from build123d import *

# Parameters (mm, degrees)
MATRIZC1_COUNT = 3


with BuildPart() as part:
    # Croquis8 → Revolución4 (revolve)
    with BuildSketch(Plane.XY):
        with BuildLine():
            Line((-10, 22.912878475), (-10, 17.320508076))
            ThreePointArc((-10, 17.320508076), (-2.679491924, 10), (0, 0))
            Line((0, 0), (10, 0))
            Line((10, 0), (10, 22.912878475))
            ThreePointArc((10, 22.912878475), (0, 25), (-10, 22.912878475))
        make_face()
    revolve(axis=Axis((0, 0, 0), (1, 0, 0)))

    # Croquis3 → Revolución5 (revolve)
    with BuildSketch(Plane(origin=(0, 0, 0), x_dir=(0, 0, -1), z_dir=(1, 0, 0))):
        with BuildLine():
            Line((0, 25), (0, 34))
            ThreePointArc((0, 34), (3.968118785, 30.50401717), (1, 26.127016654))
            Line((1, 26.127016654), (1, 24.979991994))
            ThreePointArc((1, 24.979991994), (0.50010007, 24.994997498), (0, 25))
        make_face()
    revoluci_n5 = revolve(axis=Axis((0, 25, 0), (0, 1, 0)))

    # MatrizC1: Revolución5 ×3 about axis
    matrizc1_axis = Axis((0, 0, 0), (1, 0, 0))
    for i in range(1, MATRIZC1_COUNT):
        add(revoluci_n5.rotate(matrizc1_axis, i * 360 / MATRIZC1_COUNT))


solid = part.part
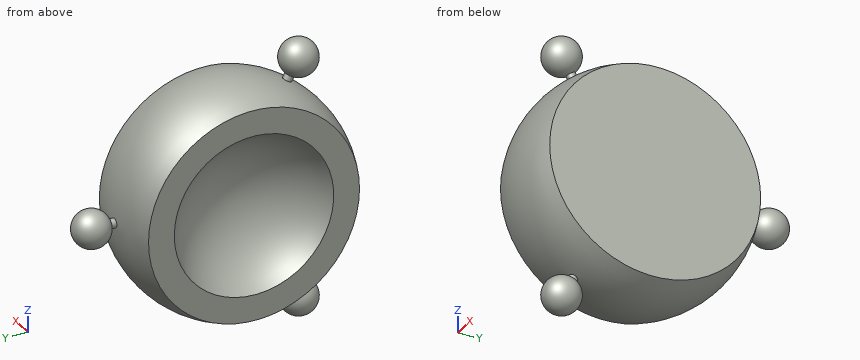
The listing builds one solid part. Answer for the finished solid, in the listing's coordinates (mm). Give positions to 0.01 mm unless a question says otherwise; leave off trailing zeros. Write each loop counter-clockwise with the first axis right and the second up, starting at its lowest first coordinate (ties: lowest second). Pieces come first, ordered by that corner, then holes. Notation, with made-up numbers: (73.5, 52) - (110.5, 52) arc R19 ccw to (110.5, 67) - close; hole circle Ø9 at (-10, -21). An arc over 180 degrees is marked (long way). One line per question, with ' | ' between items. Start each with the question number.
1. Section A-A, the plane z = 0 is taken. Determine the outline of the cut face in (x, y), then the cut area to 3 significant figures.
2. Section C-C, the plane y = -3.5 is taken. Determine the outline of the cut face in (x, z).
3. Section B-B, the plane x = -3.25 is taken. Determine the outline of the cut face in (y, z), then the cut area to 3 significant figures.
4. Straight lines are drawn through the part: line 1 (X direction, y = 25.5, z = 0); line 2 (Z direction, x = -8, y = 14.5); line 3 (Y direction, x = -5, z = 5.5). For each, find the intervals that lie inside material, in ascending order.
5. Given P1, Ø8, axis at x = -4, y = 1, coming from the +Z side; P2, Ø6, axis at x = -1.5, z = 6.5, coming from the -Y side; P3, Ø8, axis at x = -4.5, y = -18, coming from the -Z side, each flat-ended and moving along its own axis, determine where each tip first touches the part or whether it passes through.
6. Section D-D, the plane x = 2 is taken. Determine the outline of the cut face in (y, z), then the cut area to 3 significant figures.
Result:
1) outline: (-10, -22.91) arc R25 ccw to (10, -22.91) - (10, 22.91) arc R25 ccw to (1, 24.98) - (1, 26.13) arc R4 ccw (long way) to (-1, 26.13) - (-1, 24.98) arc R25 ccw to (-10, 22.91) - (-10, 17.32) arc R20 cw to (-10, -17.32) - close | area: 779 mm2
2) outline: (-10, -22.64) arc R24.75 ccw to (10, -22.64) - (10, 22.64) arc R24.75 ccw to (-10, 22.64) - (-10, 16.96) arc R19.69 cw to (-10, -16.96) - close
3) outline: circle Ø49.58 at (0, 0); circle Ø4.66 at (-15, -25.98); circle Ø4.66 at (-15, 25.98); circle Ø4.66 at (30, 0); hole circle Ø21.86 at (0, 0) | area: 1,610 mm2
4) line 1: x = -1 to 1 | line 2: z = -18.73 to -6.76, 6.76 to 18.73 | line 3: y = -23.87 to -12.03, 12.03 to 23.87
5) P1: stops at z = 25 | P2: stops at y = -24.73 | P3: stops at z = -29.72
6) outline: circle Ø49.84 at (0, 0); circle Ø6.93 at (-15, -25.98); circle Ø6.93 at (-15, 25.98); circle Ø6.93 at (30, 0) | area: 2,060 mm2
